CAD build for the part. Positions are in the model's coordinates, mm. A direction names the side the tool comes from. Give positions to 0.01 mm unless a question says otherwise; leave off trailing zeros. Loops run counter-clockwise (first coordinate to the right, second up) from the corner with the lowest first, then second, coordinate; pieces in that order, holes last. Notation, with made-up numbers: (48, 49.25) -> (70, 49.25) arc R9 ccw to (70, 62.25) -> close; hole circle Ø6 at (-25, 39). An arc over 180 degrees is marked (long way). Use one line per item in the form item = value.
```python
from build123d import *

# Parameters (mm, degrees)
SKETCH1_W                       = 114.3
SKETCH1_H                       = 101.6
BASE_FLANGE2_DEPTH              = 0.7366
EDGE_FLANGE1_DEPTH              = 101.6
F_5_32_0_15625_DIAMETER_HOLE1_D = 3.96875
F_5_32_0_15625_DIAMETER_HOLE2_D = 3.96875
SKETCH13_W                      = 88.9
SKETCH13_H                      = 76.2
CUT_EXTRUDE1_DEPTH              = 156.02325632
BREAK_CORNER1_START             = 0.7366
BREAK_CORNER1_DEPTH             = 0.7366
BREAK_CORNER1_START_2           = -0.7366
BREAK_CORNER1_2_DEPTH           = 0.7366


# Read off the part's stored shape, not the designer's step: Break-Corner1
# Sheet-metal steps are written as plain solids
with BuildPart() as part:
    # Sketch1 → Base-Flange2 (new body)
    with BuildSketch(Plane(origin=(0, 0, 0), x_dir=(1, 0, 0), z_dir=(0, 1, 0))):
        with Locations((-57.15, 50.8)):
            Rectangle(SKETCH1_W, SKETCH1_H)
    extrude(amount=-BASE_FLANGE2_DEPTH)

    # Edge-Flange1 section (across the edge) → Edge-Flange1 (add)
    with BuildSketch(Plane(origin=(0.7366, 0, 0), x_dir=(-1, 0, 0), z_dir=(0, 0, -1))):
        with BuildLine():
            Line((-0.7366, 0.7366), (-0.7366, 25.4))
            Line((-0.7366, 25.4), (0, 25.4))
            Line((0, 25.4), (0, 0.7366))
            ThreePointArc((0, 0.7366), (0.215745145, 0.215745145), (0.7366, 0))
            Line((0.7366, 0), (0.7366, -0.7366))
            ThreePointArc((0.7366, -0.7366), (-0.30510971, -0.30510971), (-0.7366, 0.7366))
        make_face()
    extrude(amount=EDGE_FLANGE1_DEPTH)

    # 5/32 (0.15625) Diameter Hole1 (through all)
    with Locations(Plane(origin=(0, 0, 0), x_dir=(1, 0, 0), z_dir=(0, 1, 0))):
        with Locations((-110.2995, 4.064), (-110.2995, 97.536), (-4.0005, 97.536), (-4.0005, 4.064)):
            Hole(F_5_32_0_15625_DIAMETER_HOLE1_D / 2)

    # 5/32 (0.15625) Diameter Hole2 (through all)
    with Locations(Plane.ZY.offset(-0.7366)):
        with Locations((-34.036, 16.436061869), (-97.536, 16.436061869)):
            Hole(F_5_32_0_15625_DIAMETER_HOLE2_D / 2)

    # Sketch13 → Cut-Extrude1 (cut, through all)
    with BuildSketch(Plane(origin=(0, 0, 0), x_dir=(1, 0, 0), z_dir=(0, 1, 0))):
        with Locations((-57.15, 50.8)):
            Rectangle(SKETCH13_W, SKETCH13_H)
    extrude(amount=-CUT_EXTRUDE1_DEPTH, mode=Mode.SUBTRACT)

    # Break-Corner1 outline → Break-Corner1 (cut)
    with BuildSketch(Plane.YZ.offset(BREAK_CORNER1_START)):
        with BuildLine():
            Line((25.4, 0), (22.86, 0))
            ThreePointArc((22.86, 0), (24.656051224, -0.743948776), (25.4, -2.54))
            Line((25.4, -2.54), (25.4, 0))
        make_face()
        with BuildLine():
            Line((25.4, -101.6), (25.4, -99.06))
            ThreePointArc((25.4, -99.06), (24.656051224, -100.856051224), (22.86, -101.6))
            Line((22.86, -101.6), (25.4, -101.6))
        make_face()
    extrude(amount=BREAK_CORNER1_DEPTH, mode=Mode.SUBTRACT)

    # Break-Corner1 2 outline → Break-Corner1 2 (cut)
    with BuildSketch(Plane(origin=(0, 0, 0), x_dir=(1, 0, 0), z_dir=(0, 1, 0)).offset(BREAK_CORNER1_START_2)):
        with BuildLine():
            Line((-114.3, 101.6), (-114.3, 99.06))
            ThreePointArc((-114.3, 99.06), (-113.556051224, 100.856051224), (-111.76, 101.6))
            Line((-111.76, 101.6), (-114.3, 101.6))
        make_face()
        with BuildLine():
            ThreePointArc((-111.76, 0), (-113.556051224, 0.743948776), (-114.3, 2.54))
            Line((-114.3, 2.54), (-114.3, 0))
            Line((-114.3, 0), (-111.76, 0))
        make_face()
    extrude(amount=BREAK_CORNER1_2_DEPTH, mode=Mode.SUBTRACT)


solid = part.part
```
1. Drop flat-ended pins along their axis: P1, Ø6, axis at y = 17.5, z = -54.5, coming from the -X side; P2, Ø3, axis at x = -4, z = -97.54, coming from the -Y side; P3, Ø12, axis at x = -33, y = 3, coming from the +Z side; P4, Ø0.8, axis at y = -0.5, z = -33.5, coming from the +X side. Give the stop position or say it passes through.
Result sheet:
P1 = 0.74
P2 = through
P3 = 0
P4 = 1.21
2. Cut at C-C, the plane z = -10.5. Write the cut outline in (x, y).
Result sheet:
outline = (-114.3, -0.74) -> (0, -0.74) arc R1.47 ccw to (1.47, 0.74) -> (1.47, 25.4) -> (0.74, 25.4) -> (0.74, 0.74) arc R0.74 cw to (0, 0) -> (-114.3, 0) -> close
3. Cut at A-A, the plane z = -72. Write the cut outline in (x, y), then the cut area to 3 significant figures.
Result sheet:
outline = (-114.3, -0.74) -> (-101.6, -0.74) -> (-101.6, 0) -> (-114.3, 0) -> close; (-12.7, -0.74) -> (0, -0.74) arc R1.47 ccw to (1.47, 0.74) -> (1.47, 25.4) -> (0.74, 25.4) -> (0.74, 0.74) arc R0.74 cw to (0, 0) -> (-12.7, 0) -> close
area = 38.2 mm^2
4. Tool access for faces 5 (the cylindrical face through (-113.536, -0.373, -0.724)), 6 (the flat face through (0.737, 13, -50)): list every direction of +Z, -Z, +X, -X, +Y, -Y with a clear straight run to the whole face (end or side of a thin tool).
Result sheet:
face_5 = +Z, -X, +Y, -Y
face_6 = +Z, -Z, -X, +Y
5. Drill centre lines: line 1 (Y direction, x = -106.5, z = -11); line 2 (X direction, y = 7, z = -25). Where is each one in solid material? Low to high.
Result sheet:
line_1 = -0.74 to 0
line_2 = 0.74 to 1.47
6. Cut at D-D, the plane y = 7.75. Write the cut outline in (x, z), then the cut area to 3 significant figures.
Result sheet:
outline = (0.74, -101.6) -> (1.47, -101.6) -> (1.47, 0) -> (0.74, 0) -> close
area = 74.8 mm^2
7. Cut at B-B, the plane x = -22. Write the cut outline in (y, z), then the cut area to 3 significant figures.
Result sheet:
outline = (-0.74, -101.6) -> (0, -101.6) -> (0, -88.9) -> (-0.74, -88.9) -> close; (-0.74, -12.7) -> (0, -12.7) -> (0, 0) -> (-0.74, 0) -> close
area = 18.7 mm^2
8. Mould opens along Z. For faces 1 (the cylindrical face through (1.1, 24.636, -0.724)), 2 (the flat face through (-58, 0, -6)), 3 (the cylindrical face through (-3.742, -0.373, -99.503)), 4 (the flat face through (-55.4, -0.2, -101.6)) say: pulls with the +Z half, pulls with the -Z half, needs draft (parallel to the pull), parting line crosses it, or undercut.
Result sheet:
face_1 = pulls with the +Z half
face_2 = needs draft
face_3 = undercut
face_4 = pulls with the -Z half
